Here's how the part is built. I have some questions about the finished solid (model axes, mm). A direction names the side the tool comes from. Coordinates: 2 decimals unless noted, no trailing zeros. Write each loop counter-clockwise with the first axis right and the second up, starting at its lowest first coordinate (ties: lowest second). Pieces come first, ordered by that corner, then holes.
Item 1: If we section it at D-D (x = 11): Please give me the cut outline in (y, z).
Item 2: For faces 5 (the face through (13.426, 0, 5)), 6 (the face through (-6, 6, 6.35)), 7 (the face through (1.238, 6, 3)), which set-ups out of +Z, -Z, +X, -X, +Y, -Y let a thin tool reach every point of the face, with its end or its side?
Item 3: If we section it at C-C (y = 14.5): Please give me the cut outline in (x, z).
Item 4: We'd pull the mould along Y, two halves only. Please class faces 1 (the face through (15.188, -8.952, -0.805)), 2 (the face through (23, -2, -1.587)), 3 (the face through (25, 8.255, 11)), 4 (the face through (15, -5.645, 5)): +Y half, -Y half, draft (parallel to the pull), parting line (faces both ways), or undercut.
Item 5: If I drill on line 1 (Y direction, x = 19.5, z = 14.5) (3 decimals); line 2 (Y direction, x = 22.5, z = 2.5) (3 decimals); line 3 (X direction, y = -6, z = 17), over which ranges is the centre line in solid material (lowest first)?
Item 6: I'm going to push flat-ended pins straight in: pin 1 Ø5 at (x, y) = (19.5, 13.5) entering from +Z; pin 2 Ø4.5 at (x, z) = (-7, 2) entering from +Y; pin 3 Ø8 at (x, y) = (26.5, -3) entering from +Z; pin 4 Ø2.5 at (x, z) = (14.5, 6) entering from -Y (3 decimals). Where does each tip first touch, or does it pass through?
Item 7: If we section it at B-B (y = -1): Please give me the cut outline in (x, z) (1 decimal), then the cut area to 3 significant figures.
Item 8: If we section it at A-A (z = 13): Please give me the cut outline in (x, y) (1 decimal), then the cut area to 3 significant figures.
from build123d import *

# Parameters (mm, degrees)
SKETCH1_W                       = 31.75
SKETCH1_H                       = 22.098
BOSS_EXTRUDE1_DEPTH             = 1.5875
F_32_0_116_DIAMETER_HOLE1_D     = 2.9464
F_32_0_116_DIAMETER_HOLE1_DEPTH = 25.4
F_32_0_116_DIAMETER_HOLE1_TIP   = 0.885187864
SKETCH4_W                       = 4.191
SKETCH4_H                       = 8.89
BOSS_EXTRUDE2_DEPTH             = 6.35
SKETCH4_3_W                     = 2.466272753
SKETCH4_3_H                     = 5.065857547
BOSS_EXTRUDE3_DEPTH             = 1.5875
BOSS_EXTRUDE4_DEPTH             = 6.35
SKETCH5_R                       = 3.81
BOSS_EXTRUDE5_DEPTH             = 9.398
BOSS_EXTRUDE5_DEPTH_BACK        = 13.208
SKETCH6_W                       = 3.302
SKETCH6_H                       = 11.289974084
BOSS_EXTRUDE6_DEPTH             = 9.398
SKETCH8_W                       = 25.019
SKETCH8_H                       = 16.51
BOSS_EXTRUDE7_DEPTH             = 15.875
CUT_EXTRUDE1_DEPTH              = 26.019
SKETCH10_W                      = 35.562788841
SKETCH10_H                      = 36.580807606
BOSS_EXTRUDE8_DEPTH             = 7.747


with BuildPart() as part:
    # Sketch1 → Boss-Extrude1 (new body)
    with BuildSketch(Plane.XY):
        Rectangle(SKETCH1_W, SKETCH1_H)
    extrude(amount=-BOSS_EXTRUDE1_DEPTH)

    # 32 _0.116_ Diameter Hole1
    with Locations(Plane.XY):
        with Locations((-13.716, 9.017), (13.716, -9.017), (13.716, 9.017), (-13.716, -9.017)):
            Hole(F_32_0_116_DIAMETER_HOLE1_D / 2, depth=F_32_0_116_DIAMETER_HOLE1_DEPTH)
            with Locations((0, 0, -(F_32_0_116_DIAMETER_HOLE1_DEPTH + F_32_0_116_DIAMETER_HOLE1_TIP / 2))):  # 118° drill point
                Cone(0, F_32_0_116_DIAMETER_HOLE1_D / 2, F_32_0_116_DIAMETER_HOLE1_TIP, mode=Mode.SUBTRACT)

    # Sketch4 → Boss-Extrude2 (add)
    with BuildSketch(Plane.XY):
        with Locations((-5.853947096, 6.4008)):
            Rectangle(SKETCH4_W, SKETCH4_H)
        with Locations((-0.857280044, 6.398532258)):
            Rectangle(SKETCH4_W, SKETCH4_H)
        with Locations((3.90076693, 6.4008)):
            Rectangle(SKETCH4_W, SKETCH4_H)
    extrude(amount=BOSS_EXTRUDE2_DEPTH)

    # Sketch4_3 → Boss-Extrude3 (add)
    with BuildSketch(Plane.XY):
        with Locations((-11.531344325, 3.722546838)):
            Rectangle(SKETCH4_3_W, SKETCH4_3_H)
    extrude(amount=BOSS_EXTRUDE3_DEPTH)

    # Sketch4_4 → Boss-Extrude4 (add)
    with BuildSketch(Plane.XY):
        with BuildLine():
            ThreePointArc((-13.267299215, -5.471435424), (-13.775299215, -5.979435424), (-13.267299215, -6.487435424))
            Line((-13.267299215, -6.487435424), (-13.267299215, -5.471435424))
        make_face()
        with BuildLine():
            Line((-13.267299215, -5.471435424), (-13.267299215, -6.487435424))
            ThreePointArc((-13.267299215, -6.487435424), (-12.90808897, -6.338645669), (-12.759299215, -5.979435424))
            ThreePointArc((-12.759299215, -5.979435424), (-12.90808897, -5.620225179), (-13.267299215, -5.471435424))
        make_face()
        with BuildLine():
            ThreePointArc((9.592700785, -5.471435424), (9.084700785, -5.979435424), (9.592700785, -6.487435424))
            Line((9.592700785, -6.487435424), (9.592700785, -5.471435424))
        make_face()
        with BuildLine():
            Line((9.592700785, -5.471435424), (9.592700785, -6.487435424))
            ThreePointArc((9.592700785, -6.487435424), (9.95191103, -6.338645669), (10.100700785, -5.979435424))
            ThreePointArc((10.100700785, -5.979435424), (9.95191103, -5.620225179), (9.592700785, -5.471435424))
        make_face()
    extrude(amount=BOSS_EXTRUDE4_DEPTH)

    # Sketch5 → Boss-Extrude5 (add, two sides)
    with BuildSketch(Plane(origin=(0, 0, 0), x_dir=(0, 0, -1), z_dir=(1, 0, 0))) as boss_extrude5_sk:
        with Locations((-6.35, -5.979435424)):
            Circle(SKETCH5_R)
    extrude(amount=BOSS_EXTRUDE5_DEPTH)
    extrude(boss_extrude5_sk.sketch, amount=-BOSS_EXTRUDE5_DEPTH_BACK)

    # Sketch6 → Boss-Extrude6 (add)
    with BuildSketch(Plane.XY):
        with Locations((15.076654567, 0)):
            Rectangle(SKETCH6_W, SKETCH6_H)
    extrude(amount=BOSS_EXTRUDE6_DEPTH)

    # Sketch8 → Boss-Extrude7 (add)
    with BuildSketch(Plane(origin=(16.727654567, 0, 0), x_dir=(0, 0, -1), z_dir=(1, 0, 0))):
        with Locations((-10.922, 0)):
            Rectangle(SKETCH8_W, SKETCH8_H)
    extrude(amount=BOSS_EXTRUDE7_DEPTH)

    # Sketch9 → Cut-Extrude1 (cut, through all)
    with BuildSketch(Plane.XY.offset(23.4315)):
        Polygon((18.378654567, 1.8288), (18.378654567, 0), (18.378654567, -1.8288), (32.602654567, -1.8288), (32.602654567, 1.8288), align=None)
        with BuildLine():
            Line((21.071054567, 6.5024), (32.602654567, 6.731))
            Line((32.602654567, 6.731), (32.602654567, 4.7625))
            Line((32.602654567, 4.7625), (32.602654567, 2.794))
            Line((32.602654567, 2.794), (21.071054567, 3.0226))
            Line((21.071054567, 3.0226), (21.071054567, 4.445))
            Line((21.071054567, 4.445), (20.515887863, 4.445))
            ThreePointArc((20.515887863, 4.445), (18.378654567, 4.7625), (20.515887863, 5.08))
            Line((20.515887863, 5.08), (21.071054567, 5.08))
            Line((21.071054567, 5.08), (21.071054567, 6.5024))
        make_face()
        with BuildLine():
            Line((21.071054567, -3.0226), (32.602654567, -2.794))
            Line((32.602654567, -2.794), (32.602654567, -4.7625))
            Line((32.602654567, -4.7625), (32.602654567, -6.731))
            Line((32.602654567, -6.731), (21.071054567, -6.5024))
            Line((21.071054567, -6.5024), (21.071054567, -5.08))
            Line((21.071054567, -5.08), (20.515887863, -5.08))
            ThreePointArc((20.515887863, -5.08), (18.378654567, -4.7625), (20.515887863, -4.445))
            Line((20.515887863, -4.445), (21.071054567, -4.445))
            Line((21.071054567, -4.445), (21.071054567, -3.0226))
        make_face()
    extrude(amount=-CUT_EXTRUDE1_DEPTH, mode=Mode.SUBTRACT)

    # Sketch10 → Boss-Extrude8 (add)
    with BuildSketch(Plane(origin=(32.602654567, 0, 0), x_dir=(0, 0, -1), z_dir=(1, 0, 0))):
        with Locations((-16.07996174, 0)):
            Rectangle(SKETCH10_W, SKETCH10_H)
    extrude(amount=BOSS_EXTRUDE8_DEPTH)


solid = part.part
Answer list:
1. outline: (-11.05, -1.59) - (11.05, -1.59) - (11.05, 0) - (-11.05, 0) - close
2. face 5: +Z, +Y, -Y
2. face 6: +Z, -X, +Y
2. face 7: +Z, +Y
3. outline: (32.6, -1.7) - (40.35, -1.7) - (40.35, 33.86) - (32.6, 33.86) - close
4. face 1: undercut
4. face 2: draft
4. face 3: +Y half
4. face 4: -Y half
5. line 1: y = -8.255 to -5.854, -3.671 to -1.829, 1.829 to 3.671, 5.854 to 8.255
5. line 2: y = -8.255 to -6.531, -2.994 to -1.829, 1.829 to 2.994, 6.531 to 8.255
5. line 3: x = 16.73 to 21.07, 32.6 to 40.35
6. pin 1: passes through
6. pin 2: stops at y = 11.05
6. pin 3: stops at z = 23.43
6. pin 4: stops at y = -5.645
7. outline: (-15.9, -1.6) - (15.9, -1.6) - (15.9, 0) - (16.7, 0) - (16.7, -1.6) - (18.4, -1.6) - (18.4, 23.4) - (16.7, 23.4) - (16.7, 9.4) - (13.4, 9.4) - (13.4, 0) - (-15.9, 0) - close; (32.6, -1.7) - (40.3, -1.7) - (40.3, 33.9) - (32.6, 33.9) - close
7. area: 398 mm2
8. outline: (16.7, -8.3) - (32.6, -8.3) - (32.6, -18.3) - (40.3, -18.3) - (40.3, 18.3) - (32.6, 18.3) - (32.6, 8.3) - (16.7, 8.3) - close; hole (18.4, -1.8) - (32.6, -1.8) - (32.6, 1.8) - (18.4, 1.8) - close; hole (20.5, -5.1) - (21.1, -5.1) - (21.1, -6.5) - (32.6, -6.7) - (32.6, -2.8) - (21.1, -3) - (21.1, -4.4) - (20.5, -4.4) arc R1.1 ccw (long way) to start; hole (20.5, 4.4) - (21.1, 4.4) - (21.1, 3) - (32.6, 2.8) - (32.6, 6.7) - (21.1, 6.5) - (21.1, 5.1) - (20.5, 5.1) arc R1.1 ccw (long way) to start
8. area: 400 mm2
